```python
from build123d import *

# Parameters (mm, degrees)
F1_DEPTH = 25
F2_W     = 44
F2_H     = 19
F3_DEPTH = 455.2712231792


# Not quite as in the source:
# - a feature names something its author has since deleted; it is built from what else it names


with BuildPart() as f1:
    # F0 (on Right) → F1 (new body, symmetric)
    with BuildSketch(Plane.YZ):
        Polygon((1862, 545.9546269485), (2050, 607.0395298403), (2042.2745751406, 630.8159427477), (1854.2745751406, 569.7310398559), align=None)
        Polygon((2042.2745751406, 630.8159427477), (2050, 607.0395298403), (2100, 623.2855146519), (2092.2745751406, 647.0619275593), align=None)
        Polygon((2092.2745751406, 647.0619275593), (2100, 623.2855146519), (2288, 684.3704175437), (2280.2745751406, 708.1468304511), align=None)
    extrude(amount=F1_DEPTH, both=True)

    # F2 (on face) → F3 (cut, through all)
    with BuildSketch(Plane(origin=(0, 1844.6468608337, 599.3620976791), x_dir=(1, 0, 0), z_dir=(0, -0.9510565163, -0.3090169944))):
        with Locations((0, -43.6559379653)):
            Rectangle(F2_W, F2_H)
    extrude(amount=-F3_DEPTH, mode=Mode.SUBTRACT)


solid = f1.part
```
The model under review builds one solid part; all positions refer to its coordinate system, in mm. A direction names the side the tool comes from. Round coordinates to 2 decimals unless told otherwise and drop trailing zeros. Order: outer loops, then holes, each group sorted by start corner. A loop starts at its lowest first (then second) coordinate and runs counter-clockwise, first axis right, second up.
Item 1: Machinability: for faces 5 (the flat face through (-22, 2068, 626)), 6 (the flat face through (-25, 2070, 627)), which of the approach directions +Z, -Z, +X, -X, +Y, -Y give a long, thin tool a straight path to every point of the face, cutting with its end or side? Answer none if there is none.
Working result:
face 5: none
face 6: +Z, -Z, -X, +Y, -Y
Item 2: Add section A-A, the plane x = 9. State the section outline as (y, z) points, and give its area (3 significant figures).
Working result:
outline: (1854.27, 569.73) - (1855.2, 566.88) - (2281.2, 705.29) - (2280.27, 708.15) - close; (1861.07, 548.81) - (1862, 545.95) - (2288, 684.37) - (2287.07, 687.22) - close
area: 2,690 mm2
Item 3: Add section C-C, the plane y = 2016.5. State the section outline as (x, z) points.
Working result:
outline: (-25, 596.15) - (25, 596.15) - (25, 622.44) - (-25, 622.44) - close; hole (-22, 599.31) - (22, 599.31) - (22, 619.29) - (-22, 619.29) - close
Item 4: Add section D-D, the plane z = 558.5. State the section outline as (x, y) points.
Working result:
outline: (-25, 1857.92) - (-22, 1857.92) - (-22, 1890.9) - (22, 1890.9) - (22, 1857.92) - (25, 1857.92) - (25, 1900.61) - (-25, 1900.61) - close
Item 5: For pin 1 (5 mm diameter, centred on x = 12, y = 1928.5, fed in from -Z); pin 2 (2 mm diameter, centred on x = -4, y = 1953, fed in from +Z), all flat-tipped, find the tip position at first contact; note any pin that passes through.
Working result:
pin 1: stops at z = 566.75
pin 2: stops at z = 602.13
Item 6: Draft analysis for pull direction Z (two halves, no side actions). For faces 1 (the flat face through (-1.74, 2287.3, 686.52)), 2 (the flat face through (-0.308, 2065.22, 635.117)), 3 (the flat face through (25, 2070, 627)), 4 (the flat face through (-1.735, 1854.972, 567.585)), state which applies: released by +Z, released by -Z, zero draft, split by the parting line, or undercut.
Working result:
face 1: released by +Z
face 2: undercut
face 3: zero draft
face 4: released by -Z
Item 7: To check wall thickness, follow probe 1 along X at (y, z) = (2159, 665); probe 2 along Z at (x, y) = (6, 2120.5); probe 3 along Z at (x, y) = (-11.5, 2025.5). State the ranges of each line that lie inside material, in increasing order.
Working result:
probe 1: x = -25 to -22, 22 to 25
probe 2: z = 629.95 to 633.1, 653.08 to 656.23
probe 3: z = 599.08 to 602.23, 622.21 to 625.37
Item 8: Add section B-B, the plane z = 655. State the section outline as (x, y) points, and give its area (3 significant figures).
Working result:
outline: (-25, 2116.71) - (25, 2116.71) - (25, 2197.61) - (-25, 2197.61) - close; hole (-22, 2126.41) - (22, 2126.41) - (22, 2187.9) - (-22, 2187.9) - close
area: 1,340 mm2
